Geometry check sheet. Reference: the model listing, model coordinates, mm. Face numbers are marked on the shaded views. A direction names the side the tool comes from. Give positions to 0.01 mm unless a question says otherwise; leave off trailing zeros. Loops run counter-clockwise (first coordinate to the right, second up) from the corner with the lowest first, then second, coordinate; pieces in that order, holes last. Notation, with made-up numbers: (46.25, -25) - (61.25, -25) arc R18 cw to (61.25, -11) - close; hole circle Ø5 at (71, 81.25). An arc over 180 degrees is marked (long way). Use a Markdown table: item, result. Add a question column.
1. Set-up check for the marked faces 1 and 2: record each of +Z, -Z, +X, -X, +Y, -Y from which the full face is reachable in a straight line by a thin tool's end or side.
2. Cross-section at D-D on z = -32. Enter the section's corners in (x, y).
3. Draft check along X on the marked faces 3, 4, 5 and 6. Enter one of: pulls with the +X half, pulls with the -X half, needs draft (parallel to the pull), parting line crosses it, or undercut.
4. Depth check by flat-ended pin: P1, Ø12, axis at x = 60, y = 17, coming from the -Z side; P2, Ø5.5, axis at x = 59.055, z = 0, coming from the -Y side; P3, Ø10, axis at x = 86, z = 21.5, coming from the +Y side; P4, Ø1, axis at x = 30.5, y = 20.5, coming from the -Z side. Enter the tip coordinate at first touch or a pass-through.
5. Cross-section at C-C on x = 72.5. Enter the section's corners in (y, z).
6. Cross-section at A-A on z = 0. Enter the section's corners in (x, y) (3 decimals).
7. Material ranges on L1, parallel to X at y = 10, z = 37; L2, parallel to Z at x = 58.5, y = 7.75; L3, parallel to Y at x = 78.5, z = 35.5, recorded low to high.
8. Cross-section at B-B on y = 6.5. Enter the section's corners in (x, z) (3 decimals).
from build123d import *

# Parameters (mm, degrees)
SKETCH2_R           = 4.5
BOSS_EXTRUDE1_DEPTH = 5
BOSS_EXTRUDE4_DEPTH = 20
SKETCH4_R           = 2
CUT_EXTRUDE1_DEPTH  = 40


with BuildPart() as part:
    # Sketch2 → Boss-Extrude1 (new body)
    with BuildSketch(Plane(origin=(0, 0, 0), x_dir=(1, 0, 0), z_dir=(0, 1, 0))):
        with BuildLine():
            Line((30.852324511, 42.360372936), (0, 26))
            ThreePointArc((0, 26), (-26, 0), (0, -26))
            Line((0, -26), (30.852324511, -42.360372936))
            ThreePointArc((30.852324511, -42.360372936), (109.945, 0), (30.852324511, 42.360372936))
        make_face()
        with Locations(Location((0, 0, 0), (0, 0, 270))):
            Circle(SKETCH2_R, mode=Mode.SUBTRACT)
        with Locations(Location((59.055, 0, 0), (0, 0, 270))):
            Circle(SKETCH2_R, mode=Mode.SUBTRACT)
    extrude(amount=BOSS_EXTRUDE1_DEPTH)

    # Sketch3 → Boss-Extrude4 (add)
    with BuildSketch(Plane(origin=(0, 5, 0), x_dir=(1, 0, 0), z_dir=(0, 1, 0))):
        with BuildLine():
            Line((30.852324511, 42.360372936), (0, 26))
            ThreePointArc((0, 26), (-26, 0), (0, -26))
            Line((0, -26), (30.852324511, -42.360372936))
            ThreePointArc((30.852324511, -42.360372936), (109.945, 0), (30.852324511, 42.360372936))
        make_face()
        with BuildLine():
            Line((0, 21), (35.989825914, 40.084687562))
            ThreePointArc((35.989825914, 40.084687562), (105.301993768, 0), (35.989825914, -40.084687562))
            Line((35.989825914, -40.084687562), (0, -21))
            ThreePointArc((0, -21), (-21, 0), (0, 21))
        make_face(mode=Mode.SUBTRACT)
    extrude(amount=BOSS_EXTRUDE4_DEPTH)

    # Sketch4 → Cut-Extrude1 (cut)
    with BuildSketch(Plane(origin=(0, 25, 0), x_dir=(1, 0, 0), z_dir=(0, 1, 0))):
        with Locations(Location((-23.3, 0, 0), (0, 0, 270))):
            Circle(SKETCH4_R)
        with Locations(Location((107.605, 0, 0), (0, 0, 270))):
            Circle(SKETCH4_R)
        with Locations(Location((44.81184785, 46.422862213, 0), (0, 0, 270))):
            Circle(SKETCH4_R)
        with Locations(Location((44.81184785, -46.316966164, 0), (0, 0, 270))):
            Circle(SKETCH4_R)
    extrude(amount=-CUT_EXTRUDE1_DEPTH, mode=Mode.SUBTRACT)


solid = part.part
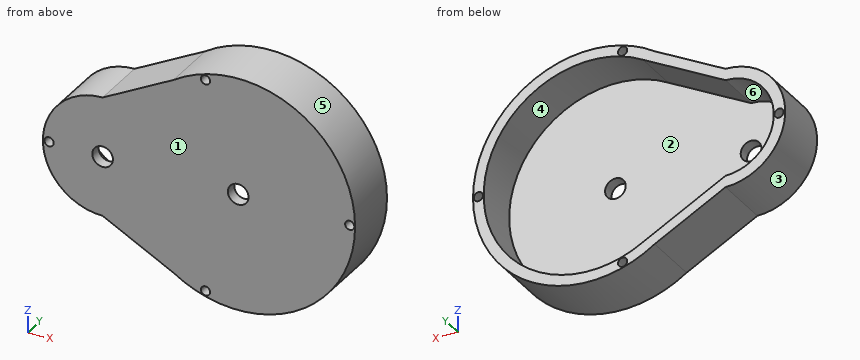
Values found:
| question | item | result |
|---|---|---|
| 1 | face 1 | +Z, -Z, +X, -X, -Y |
| 1 | face 2 | +Y |
| 2 | outline | (11.31, 0) - (98.63, 0) - (98.63, 25) - (92.44, 25) - (92.44, 5) - (20.74, 5) - (20.74, 25) - (11.31, 25) - close |
| 3 | face 3 | pulls with the -X half |
| 3 | face 4 | undercut |
| 3 | face 5 | parting line crosses it |
| 3 | face 6 | undercut |
| 4 | P1 | stops at z = -50.89 |
| 4 | P2 | passes through |
| 4 | P3 | stops at y = 5 |
| 4 | P4 | stops at z = -42.46 |
| 5 | outline | (0, -49.08) - (25, -49.08) - (25, -44.25) - (5, -44.25) - (5, 44.25) - (25, 44.25) - (25, 49.08) - (0, 49.08) - close |
| 6 | outline | (-26, 0) - (-25.3, 0) - (-25.3, 25) - (-26, 25) - close; (-21.3, 0) - (-4.5, 0) - (-4.5, 5) - (-21, 5) - (-21, 25) - (-21.3, 25) - close; (4.5, 0) - (54.555, 0) - (54.555, 5) - (4.5, 5) - close; (63.555, 0) - (105.605, 0) - (105.605, 25) - (105.302, 25) - (105.302, 5) - (63.555, 5) - close; (109.605, 0) - (109.945, 0) - (109.945, 25) - (109.605, 25) - close |
| 7 | L1 | x = 20.74 to 30.17, 86.8 to 93.99 |
| 7 | L2 | z = -50.89 to -46.24, 46.24 to 50.89 |
| 7 | L3 | y = 0 to 5 |
| 8 | outline | (0, -26) - (30.852, -42.36) arc R50.89 ccw (long way) to (30.852, 42.36) - (0, 26) arc R26 ccw to start; hole circle Ø4 at (-23.3, 0); hole (0, -21) - (35.99, -40.085) arc R46.247 ccw (long way) to (35.99, 40.085) - (0, 21) arc R21 ccw to start; hole circle Ø4 at (44.812, -46.423); hole circle Ø4 at (44.812, 46.317); hole circle Ø4 at (107.605, 0) |
